```python
from build123d import *

# Parameters (mm, degrees)
SKETCH2_R           = 5
BOSS_EXTRUDE1_DEPTH = 6.75
CUT_EXTRUDE2_DEPTH  = 1.75
FILLET1_R           = 1
CUT_EXTRUDE4_DEPTH  = 1
FILLET2_R           = 0.5
FILLET3_R           = 0.5
SKETCH10_R          = 6
BOSS_EXTRUDE2_DEPTH = 29
SKETCH11_R          = 2.5
CUT_EXTRUDE6_DEPTH  = 20


with BuildPart() as part:
    # Sketch2 → Boss-Extrude1 (new body)
    with BuildSketch(Plane(origin=(0, 0, 0), x_dir=(1, 0, 0), z_dir=(0, 1, 0))):
        with BuildLine():
            Line((-23.525392368, 12.9942923), (111.356089114, 8.996048515))
            ThreePointArc((111.356089114, 8.996048515), (120.089422447, 0), (111.356089114, -8.996048515))
            Line((111.356089114, -8.996048515), (-23.525392368, -12.9942923))
            ThreePointArc((-23.525392368, -12.9942923), (-36.910577553, 0), (-23.525392368, 12.9942923))
        make_face()
        with Locations(Location((111.089422447, 0, 0), (0, 0, 270))):
            Circle(SKETCH2_R, mode=Mode.SUBTRACT)
    extrude(amount=BOSS_EXTRUDE1_DEPTH)

    # Sketch6 → Cut-Extrude2 (cut)
    with BuildSketch(Plane(origin=(0, 6.75, 0), x_dir=(1, 0, 0), z_dir=(0, 1, 0))):
        Polygon((101.089422447, 0), (101.089422447, 15.957712546), (123.696181887, 15.957712546), (123.696181887, -15.662199351), (101.089422447, -15.662199351), align=None)
    extrude(amount=-CUT_EXTRUDE2_DEPTH, mode=Mode.SUBTRACT)

    # Fillet1
    fillet1_edges = [part.edges().sort_by_distance(p)[0] for p in [
        (101.089422447, 5.875, -9.300379664),
        (101.089422447, 5.875, 9.300379664),
    ]]
    fillet(fillet1_edges, radius=FILLET1_R)

    # Sketch9 → Cut-Extrude4 (cut)
    with BuildSketch(Plane.XZ):
        with BuildLine():
            Line((-12.452129788, 12.666051515), (77.547870212, 9.998213524))
            ThreePointArc((77.547870212, 9.998213524), (146.089422447, 0), (77.547870212, -9.998213524))
            Line((77.547870212, -9.998213524), (-12.452129788, 12.666051515))
        make_face()
    extrude(amount=-CUT_EXTRUDE4_DEPTH, mode=Mode.SUBTRACT)

    # Fillet2
    fillet2_edges = [part.edges().sort_by_distance(p)[0] for p in [
        (32.547870212, 1, 1.333918996),
    ]]
    fillet(fillet2_edges, radius=FILLET2_R)

    # Fillet3
    fillet3_edges = [part.edges().sort_by_distance(p)[0] for p in [
        (-17.988761078, 0, 12.830171908),
        (-36.910577553, 0, 0),
        (27.011238922, 0, -11.496252912),
    ]]
    fillet(fillet3_edges, radius=FILLET3_R)

    # Sketch10 → Boss-Extrude2 (add)
    with BuildSketch(Plane(origin=(0, 6.75, 0), x_dir=(1, 0, 0), z_dir=(0, 1, 0))):
        with Locations(Location((-23.910577553, 0, 0), (0, 0, 90))):
            Circle(SKETCH10_R)
    extrude(amount=BOSS_EXTRUDE2_DEPTH)

    # Sketch11 → Cut-Extrude6 (cut)
    with BuildSketch(Plane.XZ):
        with Locations(Location((-23.910577553, 0, 0), (0, 0, 270))):
            Circle(SKETCH11_R)
    extrude(amount=-CUT_EXTRUDE6_DEPTH, mode=Mode.SUBTRACT)


solid = part.part
```
Part model, mm, in its own coordinate system. A direction names the side the tool comes from. Round coordinates to 2 decimals unless told otherwise and drop trailing zeros. Order: outer loops, then holes, each group sorted by start corner. A loop starts at its lowest first (then second) coordinate and runs counter-clockwise, first axis right, second up. Notation, with made-up numbers: M 53.25,33 L 93.25,33 A13 cw 93.25,57 Z; hole C 23,74.25 d4. An arc over 180 degrees is marked long. Answer in a Markdown table with one row per item. Add a question column.
Q1. 3-axis set-ups, long thin cutter, end or side, ignore diameter. For faces 1 (the face through (70, 1, 1)), 2 (the face through (106.208, 2.972, -1.084)), 3 (the face through (-18.053, 21.047, 1.301)), 4 (the face through (-26.35, 9.86, 0.54)), 5 (the face through (27.71, 0.14, -11.32)): which of +Z, -Z, +X, -X, +Y, -Y reach the whole face in a straight line?
Q2. Cut at A-A on y = 24.5. Give the cut face in (x, z).
Q3. Pin check, flat tips, straight feed: pin 1 (3 mm diameter, centred on y = 5.5, z = -2.5, fed in from -X); pin 2 (0.9 mm diameter, centred on y = 6, z = 2, fed in from +X); pin 3 (5.5 mm diameter, centred on x = 112, z = 2, fed in from +Y); pin 4 (1.5 mm diameter, centred on x = 65.5, z = 0, fed in from +Y). Stop position of each tip, or through.
Q4. Wall check: L1, parallel to X at y = 2.6, z = 0; L2, parallel to X at y = 13.5, z = 0; L3, parallel to Y at x = 70, z = -5. Give the ranges that are in metal, low to high. Write a range as from..to.
Q5. Cut at B-B on x = 94. Give the cut face in (y, z).
Q6. Mould opens along Z. For faces 6 (the face through (105.8, 5, -0.1)), 7 (the face through (-36.907, 3.581, 0.291)), 8 (the face through (-24, 20, 0)) say: +Z half, -Z half, draft (parallel to the pull), parting line (faces both ways), or undercut.
Q7. Cut at C-C on y = 12.5. Give the cut face in (x, z), and give its area (3 significant figures).
Established:
| question | item | result |
|---|---|---|
| 1 | face 1 | +Z, +X, -Y |
| 1 | face 2 | +Y, -Y |
| 1 | face 3 | +Y |
| 1 | face 4 | -Y |
| 1 | face 5 | -Z, +X, -Y |
| 2 | outline | C -23.91,0 d12 |
| 3 | pin 1 | stops at x = -36.87 |
| 3 | pin 2 | stops at x = 101.09 |
| 3 | pin 3 | passes through |
| 3 | pin 4 | stops at y = 6.75 |
| 4 | L1 | x = -36.91..-26.41, -21.41..106.09, 116.09..120.09 |
| 4 | L2 | x = -29.91..-26.41, -21.41..-17.91 |
| 4 | L3 | y = 1..6.75 |
| 5 | outline | M 1,-9.51 L 6.75,-9.51 L 6.75,9.51 L 1,9.51 Z |
| 6 | face 6 | draft |
| 6 | face 7 | parting line |
| 6 | face 8 | undercut |
| 7 | outline | C -23.91,0 d12; hole C -23.91,0 d5 |
| 7 | area | 93.5 mm2 |
